from build123d import *

# Parameters (mm, degrees)
FUNNEL_RIGHT_SIDE_DEPTH = 155
FILLET2_R               = 10
FILLET3_R               = 2.5


with BuildPart() as part:
    # Sketch1 → Funnel - Right Side (new body)
    with BuildSketch(Plane.XY):
        with BuildLine():
            Line((0, 0), (0, 93.9))
            Line((0, 93.9), (41.974030913, 143.922702136))
            Line((41.974030913, 143.922702136), (36.974030913, 143.922702136))
            Line((36.974030913, 143.922702136), (-30, 64.106160185))
            Line((-30, 64.106160185), (-5, 32.881170193))
            Line((-5, 32.881170193), (-5, 3.266851564))
            ThreePointArc((-5, 3.266851564), (-2.484755158, 1.656758403), (0, 0))
        make_face()
    extrude(amount=FUNNEL_RIGHT_SIDE_DEPTH)

    # Fillet2
    fillet2_edges = [part.edges().sort_by_distance(p)[0] for p in [
        (-5, 32.881170193, 77.5),
        (0, 93.9, 77.5),
    ]]
    fillet(fillet2_edges, radius=FILLET2_R)

    # Fillet3
    fillet3_edges = [part.edges().sort_by_distance(p)[0] for p in [
        (-30, 64.106160185, 77.5),
    ]]
    fillet(fillet3_edges, radius=FILLET3_R)


solid = part.part
Can you work these out from the model? Positions are in its coordinate system, mm. A direction names the side the tool comes from. Round coordinates to 2 decimals unless told otherwise and drop trailing zeros. Loops run counter-clockwise (first coordinate to the right, second up) from the corner with the lowest first, then second, coordinate; pieces in that order, holes last. Notation, with made-up numbers: (55.5, 16.25) - (93.5, 16.25) arc R23 cw to (93.5, 31.25) - close; hole circle Ø9 at (44, 2). An arc over 180 degrees is marked (long way). Write item = value, one per line. Start each with the question number.
(1) If we section it at B-B (y = 19): Please give me the cut outline in (x, z).
(2) For P1, Ø12, axis at x = 33.5, z = 115.5, coming from the -Y side; P2, Ø10, axis at y = 107.5, z = 60, coming from the +X side; P3, Ø21, axis at y = 12, z = 96.5, coming from the -X side, each with a flat end and sliding along its axis, tell me the tip position at first contact or that it passes through.
(3) If we section it at C-C (x = -16.5): Please give me the cut outline in (y, z), and give its area (3 significant figures).
(4) For faces 1 (the face through (4.61, 105.35, 76.41)), 2 (the face through (-5, 17, 76)), 3 (the face through (0, 44, 76)), which set-ups out of +Z, -Z, +X, -X, +Y, -Y let a thin tool reach every point of the face, with its end or its side?
(5) If we section it at A-A (z = 111.5): Please give me the cut outline in (x, y), and give its area (3 significant figures).
(6) If I drill on probe 1 along X at (y, z) = (25, 58.5); probe 2 along X at (y, z) = (133, 98); probe 3 along Y at (x, z) = (14.5, 134.5), over which ranges is the centre line in solid material (lowest first)? Write a range as [from, to].
Ans:
q1.outline = (-5, 0) - (0, 0) - (0, 155) - (-5, 155) - close
q2.P1 = 126.67
q2.P2 = 15.61
q2.P3 = -5
q3.outline = (47.24, 0) - (80.19, 0) - (80.19, 155) - (47.24, 155) - close
q3.area = 5,110 mm²
q4.face_1 = +Z, -Z, -X, +Y
q4.face_2 = +Z, -Z, -X, -Y
q4.face_3 = +Z, -Z, +X, -Y
q5.outline = (-28.72, 62.51) - (-7.19, 35.62) arc R10 cw to (-5, 29.37) - (-5, 3.27) arc R160 cw to (0, 0) - (0, 90.26) arc R10 cw to (2.34, 96.69) - (41.97, 143.92) - (36.97, 143.92) - (-28.68, 65.68) arc R2.5 ccw to start
q5.area = 1,480 mm²
q6.probe_1 = [-5, 0]
q6.probe_2 = [27.81, 32.81]
q6.probe_3 = [111.18, 117.14]
